The model under review builds one solid part; all positions refer to its coordinate system, in mm. A direction names the side the tool comes from. Coordinates: 2 decimals unless noted, no trailing zeros. Write each loop counter-clockwise with the first axis right and the second up, starting at its lowest first coordinate (ties: lowest second). Pieces come first, ordered by that corner, then holes.
1) For line 1 (Y direction, x = 97.5, z = 1.05); line 2 (Y direction, x = -260, z = 0.9); line 3 (Y direction, x = -130, z = 0.25), list the stretches that pass through material, from the lowest coordinate up.
2) Mouldability with a two-part tool opening along Y and no side actions: class faces 4 (the flat face through (261.867, -10.138, 1.568)), 5 (the flat face through (265.016, -42.047, 1.568)), 6 (the cylindrical face through (336.624, 4.596, 1.568)), 7 (the cylindrical face through (-1.38, -6.2, 1.61)) as released by +Y, released by -Y, zero draft, split by the parting line, or undercut.
3) Add section B-B, the plane z = 0.8. Give the number of separate pieces and of enclosed holes in the cut face, then the cut area to 3 significant figures.
4) Add section D-D, the plane x = -170. State the section outline as (y, z) points.
5) For P1, Ø1.5, axis at x = 150.5, z = 2.5, coming from the -Y side; P2, Ø1, axis at y = -9.5, z = 3, coming from the -X side; P3, Ø1.5, axis at y = -39, z = 2, coming from the +X side, all flat-tipped, find the tip position at first contact; note any pin that passes through.
6) Machinability: for faces 1 (the flat face through (-5, -24, 3.18)), 2 (the flat face through (-260.198, -10.758, 1.568)), 3 (the flat face through (-97.78, -50.07, 1.57)), which of the approach directions +Z, -Z, +X, -X, +Y, -Y give a long, thin tool a straight path to every point of the face, cutting with its end or side? Answer none if there is none.
7) Add section C-C, the plane x = -271. State the section outline as (y, z) points, then the cut area to 3 significant figures.
8) Add section A-A, the plane y = -48. State the section outline as (x, z) points.
from build123d import *

# Parameters (mm, degrees)
BOSS_EXTRUDE1_DEPTH = 3.18
SKETCH2_R           = 6.35
SKETCH2_R_2         = 3.175
SKETCH2_R_3         = 1.65
CUT_EXTRUDE1_DEPTH  = 4.18


with BuildPart() as part:
    # Sketch1 → Boss-Extrude1 (new body)
    with BuildSketch(Plane.XY):
        with BuildLine():
            Line((-7.486391976, 23.852755295), (-188.46282125, -32.948250341))
            ThreePointArc((-188.46282125, -32.948250341), (-194.970418947, -33.859324331), (-201.422047732, -32.612179737))
            Line((-201.422047732, -32.612179737), (-320.643679437, 11.71633352))
            ThreePointArc((-320.643679437, 11.71633352), (-336.523287364, 4.843949662), (-330.323051891, -11.309956612))
            Line((-330.323051891, -11.309956612), (-201.512349729, -71.934950616))
            ThreePointArc((-201.512349729, -71.934950616), (-194.881579427, -73.749885885), (-188.027959697, -73.212297358))
            Line((-188.027959697, -73.212297358), (-4.967507005, -26.273719745))
            ThreePointArc((-4.967507005, -26.273719745), (0, -25.646997066), (4.967507005, -26.273719745))
            Line((4.967507005, -26.273719745), (188.027959697, -73.212297358))
            ThreePointArc((188.027959697, -73.212297358), (194.881579427, -73.749885885), (201.512349729, -71.934950616))
            Line((201.512349729, -71.934950616), (330.323051891, -11.309956612))
            ThreePointArc((330.323051891, -11.309956612), (336.523287364, 4.843949662), (320.643679437, 11.71633352))
            Line((320.643679437, 11.71633352), (201.422047732, -32.612179737))
            ThreePointArc((201.422047732, -32.612179737), (194.970418947, -33.859324331), (188.46282125, -32.948250341))
            Line((188.46282125, -32.948250341), (7.486391976, 23.852755295))
            ThreePointArc((7.486391976, 23.852755295), (0, 25), (-7.486391976, 23.852755295))
        make_face()
    extrude(amount=BOSS_EXTRUDE1_DEPTH)

    # Sketch2 → Cut-Extrude1 (cut, through all)
    with BuildSketch(Plane.XY.offset(3.18)):
        Circle(SKETCH2_R)
        with Locations((-325, 0)):
            Circle(SKETCH2_R_2)
        with Locations((-97.5, -11.398788164)):
            Circle(SKETCH2_R_3)
        with Locations((-195, -66.738312644)):
            Circle(SKETCH2_R_3)
        with Locations((-260, -17.831958341)):
            Circle(SKETCH2_R_3)
        with Locations((97.5, -11.398788164)):
            Circle(SKETCH2_R_3)
        with Locations((195, -66.738312644)):
            Circle(SKETCH2_R_3)
        with Locations((260, -17.831958341)):
            Circle(SKETCH2_R_3)
        with Locations((325, 0)):
            Circle(SKETCH2_R_2)
    extrude(amount=-CUT_EXTRUDE1_DEPTH, mode=Mode.SUBTRACT)


solid = part.part
Geometry results:
1. line 1: y = -50 to -13.05, -9.75 to -4.4
1. line 2: y = -44.41 to -19.48, -16.18 to -10.83
1. line 3: y = -58.33 to -14.6
2. face 4: released by +Y
2. face 5: released by -Y
2. face 6: split by the parting line
2. face 7: undercut
3. separate pieces: 1
3. enclosed holes: 9
3. area: 26,800 mm2
4. outline: (-68.59, 0) - (-27.15, 0) - (-27.15, 3.18) - (-68.59, 3.18) - close
5. P1: stops at y = -63.78
5. P2: stops at x = -333.67
5. P3: stops at x = 273.08
6. face 1: +Z, +X, -X, +Y, -Y
6. face 2: +Z, -Z, +Y
6. face 3: +Z, -Z, -Y
7. outline: (-39.23, 0) - (-6.74, 0) - (-6.74, 3.18) - (-39.23, 3.18) - close
7. area: 103 mm2
8. outline: (-252.37, 0) - (-89.7, 0) - (-89.7, 3.18) - (-252.37, 3.18) - close; (89.7, 0) - (252.37, 0) - (252.37, 3.18) - (89.7, 3.18) - close
